Model file for the job. Use its own axes, mm. Round coordinates to 2 decimals unless told otherwise and drop trailing zeros. Loops run counter-clockwise (first coordinate to the right, second up) from the corner with the lowest first, then second, coordinate; pieces in that order, holes last. Notation, with made-up numbers: M -0.5,29.5 L 44.5,29.5 A25 ccw 44.5,49.5 Z; hole C 26,69 d6. An arc over 180 degrees is marked long. Use a Markdown table: item, result. Add a question column.
Item 1: Saw through at A-A on x = -21. Write the cut outline in (y, z), then the cut area to 3 significant figures.
Item 2: Saw through at D-D on x = 7.5. Write the cut outline in (y, z).
Item 3: Pin check, flat tips, straight feed: P1, Ø4, axis at y = -4, z = -6.5, coming from the +X side; P2, Ø1.5, axis at y = -1, z = 4.5, coming from the +X side; P3, Ø2, axis at x = 16, y = -5.5, coming from the -Z side; P4, Ø11.5, axis at x = 0, z = 0, coming from the -Y side. Stop position of each tip, or through.
Item 4: Saw through at B-B on y = -4.75. Write the cut outline in (x, z) (3 decimals).
Item 5: Two-plate mould, pull along X, no slides. Class faces 1 (the flat face through (0, 0, -5)), 2 (the cylindrical face through (-0.579, -3.757, -13.373)): +X half, -X half, draft (parallel to the pull), parting line (faces both ways), or undercut.
Item 6: Saw through at C-C on z = -17.78. Write the cut outline in (x, y) (3 decimals).
Item 7: Wall check: L1, parallel to Z at x = 18.5, y = -7.25; L2, parallel to Z at x = 16, y = -2.25; L3, parallel to X at y = -3.5, z = 20.5. Give the ranges that are in metal, low to high. Write a range as from..to.
```python
from build123d import *

# Parameters (mm, degrees)
F0_R     = 4.445
F1_DEPTH = 7.62


# Not quite as in the source:
# - a feature names something its author has since deleted; it is built from what else it names


with BuildPart() as f1:
    # F0 (on Front) → F1 (new body)
    with BuildSketch(Plane.XZ):
        with BuildLine():
            Line((6.35, 17.78), (6.35, 6.35))
            Line((6.35, 6.35), (17.78, 6.35))
            ThreePointArc((17.78, 6.35), (22.2701280605, 4.4901280605), (24.13, 0))
            ThreePointArc((24.13, 0), (17.06248663, 17.06248663), (0, 24.13))
            ThreePointArc((0, 24.13), (4.4901280605, 22.2701280605), (6.35, 17.78))
        make_face()
        with BuildLine():
            Line((17.78, -6.35), (6.35, -6.35))
            Line((6.35, -6.35), (6.35, -17.78))
            ThreePointArc((6.35, -17.78), (4.4901280329, -22.2701280882), (-7.83e-08, -24.13))
            ThreePointArc((-7.83e-08, -24.13), (17.0624866024, -17.0624866577), (24.13, 0))
            ThreePointArc((24.13, 0), (22.2701280605, -4.4901280605), (17.78, -6.35))
        make_face()
        with BuildLine():
            Line((-17.78, 6.35), (-6.35, 6.35))
            Line((-6.35, 6.35), (-6.35, 17.78))
            ThreePointArc((-6.35, 17.78), (-4.4901280605, 22.2701280605), (0, 24.13))
            ThreePointArc((0, 24.13), (-17.0624866246, 17.0624866355), (-24.13, 1.54e-08))
            ThreePointArc((-24.13, 1.54e-08), (-22.2701280551, 4.490128066), (-17.78, 6.35))
        make_face()
        with BuildLine():
            Line((-6.35, -17.78), (-6.35, -6.35))
            Line((-6.35, -6.35), (-17.78, -6.35))
            ThreePointArc((-17.78, -6.35), (-22.270128066, -4.4901280551), (-24.13, 1.54e-08))
            ThreePointArc((-24.13, 1.54e-08), (-17.0624866631, -17.0624865969), (-7.83e-08, -24.13))
            ThreePointArc((-7.83e-08, -24.13), (-4.4901280882, -22.2701280329), (-6.35, -17.78))
        make_face()
        with BuildLine():
            ThreePointArc((-6.35, 17.78), (0, 11.43), (6.35, 17.78))
            ThreePointArc((6.35, 17.78), (4.4901280605, 22.2701280605), (0, 24.13))
            ThreePointArc((0, 24.13), (-4.4901280605, 22.2701280605), (-6.35, 17.78))
        make_face()
        with Locations((0, 17.78)):
            Circle(F0_R, mode=Mode.SUBTRACT)
        with BuildLine():
            ThreePointArc((24.13, 0), (22.2701280605, 4.4901280605), (17.78, 6.35))
            ThreePointArc((17.78, 6.35), (11.43, 0), (17.78, -6.35))
            ThreePointArc((17.78, -6.35), (22.2701280605, -4.4901280605), (24.13, 0))
        make_face()
        with Locations((17.78, 0)):
            Circle(F0_R, mode=Mode.SUBTRACT)
        with BuildLine():
            ThreePointArc((-7.83e-08, -24.13), (4.4901280329, -22.2701280882), (6.35, -17.78))
            ThreePointArc((6.35, -17.78), (0, -11.43), (-6.35, -17.78))
            ThreePointArc((-6.35, -17.78), (-4.4901280882, -22.2701280329), (-7.83e-08, -24.13))
        make_face()
        with Locations((0, -17.78)):
            Circle(F0_R, mode=Mode.SUBTRACT)
        with BuildLine():
            ThreePointArc((-11.43, 0), (-13.2898719395, 4.4901280605), (-17.78, 6.35))
            ThreePointArc((-17.78, 6.35), (-22.2701280551, 4.490128066), (-24.13, 1.54e-08))
            ThreePointArc((-24.13, 1.54e-08), (-22.270128066, -4.4901280551), (-17.78, -6.35))
            ThreePointArc((-17.78, -6.35), (-13.2898719395, -4.4901280605), (-11.43, 0))
        make_face()
        with Locations((-17.78, 0)):
            Circle(F0_R, mode=Mode.SUBTRACT)
        with BuildLine():
            ThreePointArc((0, -6.35), (4.4901280605, -4.4901280605), (6.35, 0))
            ThreePointArc((6.35, 0), (4.4901280605, 4.4901280605), (0, 6.35))
            ThreePointArc((0, 6.35), (-4.4901280605, 4.4901280605), (-6.35, 0))
            ThreePointArc((-6.35, 0), (-4.4901280605, -4.4901280605), (0, -6.35))
        make_face()
        Circle(F0_R, mode=Mode.SUBTRACT)
        with BuildLine():
            ThreePointArc((-6.35, 0), (-4.4901280605, 4.4901280605), (0, 6.35))
            Line((0, 6.35), (-6.35, 6.35))
            Line((-6.35, 6.35), (-6.35, 0))
        make_face()
        with BuildLine():
            Line((-6.35, -6.35), (0, -6.35))
            ThreePointArc((0, -6.35), (-4.4901280605, -4.4901280605), (-6.35, 0))
            Line((-6.35, 0), (-6.35, -6.35))
        make_face()
        with BuildLine():
            Line((6.35, -6.35), (6.35, 0))
            ThreePointArc((6.35, 0), (4.4901280605, -4.4901280605), (0, -6.35))
            Line((0, -6.35), (6.35, -6.35))
        make_face()
        with BuildLine():
            ThreePointArc((0, 6.35), (4.4901280605, 4.4901280605), (6.35, 0))
            Line((6.35, 0), (6.35, 6.35))
            Line((6.35, 6.35), (0, 6.35))
        make_face()
        with BuildLine():
            Line((-6.35, -6.35), (-6.35, 0))
            Line((-6.35, 0), (-6.35, 6.35))
            Line((-6.35, 6.35), (-17.78, 6.35))
            ThreePointArc((-17.78, 6.35), (-13.2898719395, 4.4901280605), (-11.43, 0))
            ThreePointArc((-11.43, 0), (-13.2898719395, -4.4901280605), (-17.78, -6.35))
            Line((-17.78, -6.35), (-6.35, -6.35))
        make_face()
        with BuildLine():
            Line((6.35, -6.35), (0, -6.35))
            Line((0, -6.35), (-6.35, -6.35))
            Line((-6.35, -6.35), (-6.35, -17.78))
            ThreePointArc((-6.35, -17.78), (0, -11.43), (6.35, -17.78))
            Line((6.35, -17.78), (6.35, -6.35))
        make_face()
        with BuildLine():
            Line((6.35, 6.35), (6.35, 0))
            Line((6.35, 0), (6.35, -6.35))
            Line((6.35, -6.35), (17.78, -6.35))
            ThreePointArc((17.78, -6.35), (11.43, 0), (17.78, 6.35))
            Line((17.78, 6.35), (6.35, 6.35))
        make_face()
        with BuildLine():
            Line((-6.35, 6.35), (0, 6.35))
            Line((0, 6.35), (6.35, 6.35))
            Line((6.35, 6.35), (6.35, 17.78))
            ThreePointArc((6.35, 17.78), (0, 11.43), (-6.35, 17.78))
            Line((-6.35, 17.78), (-6.35, 6.35))
        make_face()
    extrude(amount=F1_DEPTH)


solid = f1.part
```
Entries:
| question | item | result |
|---|---|---|
| 1 | outline | M -7.62,-11.89 L 0,-11.89 L 0,-3.06 L -7.62,-3.06 Z; M -7.62,3.06 L 0,3.06 L 0,11.89 L -7.62,11.89 Z |
| 1 | area | 134 mm2 |
| 2 | outline | M -7.62,-22.93 L 0,-22.93 L 0,22.93 L -7.62,22.93 Z |
| 3 | P1 | x = 23.71 |
| 3 | P2 | x = 23.84 |
| 3 | P3 | z = -18.9 |
| 3 | P4 | y = -7.62 |
| 4 | outline | C 0,0 d48.26; hole C -17.78,0 d8.89; hole C 0,-17.78 d8.89; hole C 0,0 d8.89; hole C 0,17.78 d8.89; hole C 17.78,0 d8.89 |
| 5 | face 1 | draft |
| 5 | face 2 | undercut |
| 6 | outline | M -16.313,-7.62 L -4.445,-7.62 L -4.445,0 L -16.313,0 Z; M 4.445,-7.62 L 16.313,-7.62 L 16.313,0 L 4.445,0 Z |
| 7 | L1 | -15.49..-4.39, 4.39..15.49 |
| 7 | L2 | -18.06..-4.07, 4.07..18.06 |
| 7 | L3 | -12.73..-3.52, 3.52..12.73 |
